Autodesk Fusion 360 part; units mm, degrees
sketch "Sketch1" plane through (0, 0, 0) normal (0, 0, 1) x (1, 0, 0)
  line L0 (0, 0) -> (16, 0)
  line L1 (16, 0) -> (16, 2)
  line L2 (16, 2) -> (2, 2)
  line L3 (2, 2) -> (2, 16)
  line L4 (2, 16) -> (0, 16)
  line L5 (0, 16) -> (0, 0)
  dimension "d1" = 16
  dimension "d2" = 16
  dimension "d3" = 2
  dimension "d4" = 2
extrude "Extrude1" add sketch "Sketch1" against normal blind 46
sketch "Sketch2" plane through (0, 2, 0) normal (0, 1, 0) x (-1, 0, 0)
  line L0 (-2, 0) -> (-16, 0)
  line L1 (-16, 0) -> (-16, -46)
  line L2 (-16, -46) -> (-2, -46)
  line L3 (-2, -46) -> (-2, 0)
  line L4 (-9, -46) -> (-9, 0) construction
  line L5 (-16, -23) -> (-2, -23) construction
  circle A0 centre (-9, -10.3) radius 2.5
  circle A1 centre (-9, -35.7) radius 2.5
  dimension "d7" = 5
  dimension "d19" = 12.7
extrude "Extrude2" cut sketch "Sketch2" against normal blind 2 contours A0 | A1
sketch "Sketch3" plane through (2, 0, 0) normal (1, 0, 0) x (0, 0, -1)
  line L0 (0, 16) -> (0, 2)
  line L1 (0, 2) -> (46, 2)
  line L2 (46, 2) -> (46, 16)
  line L3 (46, 16) -> (0, 16)
  line L4 (23, 16) -> (23, 2) construction
  line L5 (0, 9) -> (46, 9) construction
  circle A0 centre (7, 9) radius 3.2
  line L6 (0, 12.2) -> (46, 12.2) construction
  line L7 (0, 6.2) -> (46, 6.2) construction
  line L8 (5.4508, 6.2) -> (8.5492, 6.2)
  circle A1 centre (39, 9) radius 3.2
  line L9 (40.5492, 6.2) -> (37.4508, 6.2)
  dimension "d10" = 6.4
  dimension "d11" = 6
  dimension "d12" = 16
extrude "Extrude3" cut sketch "Sketch3" against normal blind 2 contours A0 L8 | A1 L9 picked at (6.9734, 8.1997) picked at (38.4662, 7.5792)
fillet "Fillet1" radius 2 1 edges at (2, 2, -23)
fillet "Fillet2" radius 3 4 edges at (1, 16, -46) (1, 16, 0) (16, 1, 0) (16, 1, -46)
equation "d12 = ( 32 / 2 ) * 1 mm"
equation "d19 = ( 25.4 / 2 ) * 1 mm"
Input: part model. Units: mm. Frame: model coordinates. A direction names the side the tool comes from. Give positions to 0.01 mm unless a question says otherwise; leave off trailing zeros. Write each loop counter-clockwise with the first axis right and the second up, starting at its lowest first coordinate (ties: lowest second). Pieces come first, ordered by that corner, then holes. Notation, with made-up numbers: (-16, 31) - (-9, 31) arc R14 ccw to (-9, 49) - close; hole circle Ø1 at (16.5, 34). An arc over 180 degrees is marked (long way). Write item = value, one per line. Start each with the question number.
1. Ray query, L1, parallel to Z at x = 1.15, y = 9; L2, parallel to Z at x = 9, y = 0.6; L3, parallel to X at y = 11, z = -24.5. Return the intervals inside material, ascending.
2. Section query D-D, the plane y = 1.5. Output: boundary loops of the cut face in (x, z), then the cut area to 3 significant figures.
3. Section query B-B, the plane x = 7.5. Output: boundary loops of the cut face in (y, z).
4. Access query for faces 1 (the flat face through (1, 6.2, -39)), 2 (the cylindrical face through (15.14, 1.01, -45.1)), 3 (the flat face through (2, 10, -23)). Directions: +Z, -Z, +X, -X, +Y, -Y. A direction counts if a zero-diameter tool reaches every point of the face in a straight line with its end or side. Return the directions, or none.
5. Section query C-C, the plane z = -26. Output: boundary loops of the cut face in (x, y), then the cut area to 3 significant figures.
6. Mould query, pull axis Z, two halves, no side actions, for faces 4 (the cylindrical face through (0.99, 15.14, -45.1)), 5 (the cylindrical face through (1, 12.2, -39.1)), 6 (the cylindrical face through (0.99, 15.1, -0.86)), 7 (the flat face through (10, 2, -23)). Classes: released by +Z, released by -Z, zero draft, split by the parting line, or undercut.
7. Section query A-A, the plane y = 9. Output: boundary loops of the cut face in (x, z).
8. First-contact query: pin 1 Ø1.5 at (x, y) = (4.5, 7) entering from -Z; pin 2 Ø4 at (y, z) = (14, -35) entering from +X; pin 3 Ø1 at (y, z) = (4, -39) entering from +X; pin 4 Ø9.5 at (x, z) = (10, -14) entering from +Y. Flat tips, straight axial feed; report the tip coordinate or a pass-through.
Check sheet entries:
q1.L1 = -46 to -42.2, -35.8 to -10.2, -3.8 to 0
q1.L2 = -46 to -38.2, -33.2 to -12.8, -7.8 to 0
q1.L3 = 0 to 2
q2.outline = (0, -46) - (13, -46) arc R3 ccw to (16, -43) - (16, -3) arc R3 ccw to (13, 0) - (0, 0) - close; hole circle Ø5 at (9, -35.7); hole circle Ø5 at (9, -10.3)
q2.area = 693 mm2
q3.outline = (0, -46) - (2, -46) - (2, -37.7) - (0, -37.7) - close; (0, -33.7) - (2, -33.7) - (2, -12.3) - (0, -12.3) - close; (0, -8.3) - (2, -8.3) - (2, 0) - (0, 0) - close
q4.face_1 = +X, -X
q4.face_2 = -Z, +X, +Y, -Y
q4.face_3 = +Z, -Z, +X, +Y
q5.outline = (0, 0) - (16, 0) - (16, 2) - (4, 2) arc R2 cw to (2, 4) - (2, 16) - (0, 16) - close
q5.area = 60.9 mm2
q6.face_4 = released by -Z
q6.face_5 = undercut
q6.face_6 = released by +Z
q6.face_7 = zero draft
q7.outline = (0, -46) - (2, -46) - (2, -42.2) - (0, -42.2) - close; (0, -35.8) - (2, -35.8) - (2, -10.2) - (0, -10.2) - close; (0, -3.8) - (2, -3.8) - (2, 0) - (0, 0) - close
q8.pin_1 = through
q8.pin_2 = 2
q8.pin_3 = 2.06
q8.pin_4 = 2
